```python
from build123d import *

# Parameters (mm, degrees)
F1_DEPTH = 38
F2_W     = 324
F2_H     = 38
F3_DEPTH = 38
F4_W     = 38
F4_H     = 38
F5_DEPTH = 324
F7_DEPTH = 38
F8_T     = -2.5


with BuildPart() as f1:
    # F0 (on Front) → F1 (new body)
    with BuildSketch(Plane.XZ):
        Polygon((0, 200), (0, 0), (38, 0), (38, 162), (1162, 162), (1162, 0), (1200, 0), (1200, 200), (1162, 200), (38, 200), align=None)
    extrude(amount=F1_DEPTH)

    # F2 (on face) → F3 (join)
    with BuildSketch(Plane(origin=(0, 0, 0), x_dir=(0, -1, 0), z_dir=(-1, 0, 0))):
        with Locations((-162, 181)):
            Rectangle(F2_W, F2_H)
    extrude(amount=-F3_DEPTH)

    # F4 (on face) → F5 (join)
    with BuildSketch(Plane(origin=(0, 0, 0), x_dir=(-1, 0, 0), z_dir=(0, 1, 0))):
        with Locations((-1181, 181)):
            Rectangle(F4_W, F4_H)
    extrude(amount=F5_DEPTH)

    # F6 (on face) → F7 (join)
    with BuildSketch(Plane(origin=(0, 324, 0), x_dir=(-1, 0, 0), z_dir=(0, 1, 0))):
        Polygon((-1162, 200), (-1200, 200), (-1200, 162), (-1200, 0), (-1162, 0), (-1162, 162), (-38, 162), (-38, 0), (0, 0), (0, 162), (0, 200), (-38, 200), align=None)
    extrude(amount=F7_DEPTH)

    # F8
    f8_openings = [f1.faces().sort_by_distance(p)[0] for p in [
        (19, 343, 0),
        (19, -19, 0),
        (1181, -19, 0),
        (1181, 343, 0),
    ]]
    offset(amount=F8_T, openings=f8_openings, kind=Kind.INTERSECTION)


solid = f1.part
```
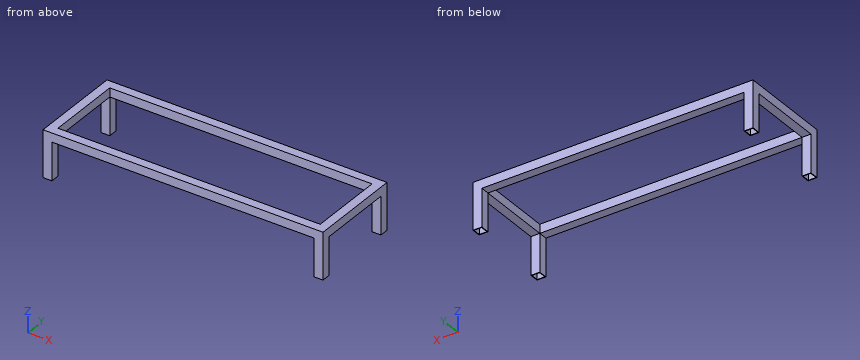
The model under review builds one solid part; all positions refer to its coordinate system, in mm. Give positions to 0.01 mm unless a question says otherwise; leave off trailing zeros. Write each loop counter-clockwise with the first axis right and the second up, starting at its lowest first coordinate (ties: lowest second). Pieces come first, ordered by that corner, then holes.
(1) To check wall thickness, follow L1, parallel to X at y = -5, z = 150.5; L2, parallel to Y at x = 1113, z = 181; L3, parallel to Z at x = 515, y = 331. State the ranges of each line that lie inside material, in increasing order.
(2) Consider section B-B, the plane z = 180.5. Give the boundary of the cut face in (x, y).
(3) Consider section A-A, the plane x = 513.5. Give the boundary of the cut face in (y, z), and give its area (3 significant figures).
(4) For P1, Ø12, axis at y = 321, z = 89.5, coming from the +X side; P2, Ø19, axis at x = 392.5, y = 344.5, coming from the -Z side, all flat-tipped, find the tip position at first contact; note any pin that passes through.
(5) Consider section C-C, the plane z = 12.5. Give the number of separate pieces and of enclosed holes in the cut face, and give its area (3 significant figures).
Returned:
1. L1: x = 0 to 2.5, 35.5 to 38, 1162 to 1164.5, 1197.5 to 1200
1. L2: y = -38 to -35.5, -2.5 to 0, 324 to 326.5, 359.5 to 362
1. L3: z = 162 to 164.5, 197.5 to 200
2. outline: (0, -38) - (1200, -38) - (1200, 362) - (0, 362) - close; (35.5, -2.5) - (1164.5, -2.5) - (1164.5, 326.5) - (35.5, 326.5) - close; hole (2.5, -35.5) - (1197.5, -35.5) - (1197.5, 359.5) - (2.5, 359.5) - close; hole (38, 0) - (1162, 0) - (1162, 324) - (38, 324) - close
3. outline: (-38, 162) - (0, 162) - (0, 200) - (-38, 200) - close; (324, 162) - (362, 162) - (362, 200) - (324, 200) - close; hole (-35.5, 164.5) - (-2.5, 164.5) - (-2.5, 197.5) - (-35.5, 197.5) - close; hole (326.5, 164.5) - (359.5, 164.5) - (359.5, 197.5) - (326.5, 197.5) - close
3. area: 710 mm2
4. P1: stops at x = 1200
4. P2: stops at z = 162
5. separate pieces: 4
5. enclosed holes: 4
5. area: 1,420 mm2
